The listing builds one solid part. Answer for the finished solid, in the listing's coordinates (mm). Face numbers are marked on the shaded views. A direction names the side the tool comes from. Give positions to 0.01 mm unless a question says otherwise; leave off trailing zeros. Loops run counter-clockwise (first coordinate to the right, second up) from the corner with the lowest first, then second, coordinate; pieces in that order, holes last. Notation, with made-up numbers: M 73.5,36 L 91.5,36 A25 cw 91.5,71 Z; hole C 7,-8 d11. An arc over 180 degrees is marked long. One line per item, written item: value. Start each with the question number.
Q1. The mould has two halves that part along X. Classify the marked faces 6, 7 and 8: +X half, -X half, draft (parallel to the pull), parting line (faces both ways), or undercut.
Q2. Consider L1, parallel to X at y = 7.5, z = 21.5; L2, parallel to Y at x = 8.5, z = 12.5. Determine where each line is inside the solid, lowest interval first.
Q3. For the marked faces 1, 2, 3, 4 and 5, determine the directions among +Z, -Z, +X, -X, +Y, -Y from which every point of the face is accessible in a straight line to the end or side of a thin tool.
Q4. Flat-ended cylindrical pins translate along their axes: pin 1 (8 mm diameter, centred on x = 4, z = 16, fed in from +Y); pin 2 (0.9 mm diameter, centred on x = 18, z = 27.5, fed in from +Y); pin 3 (3.5 mm diameter, centred on x = 1, y = 26.5, fed in from +Z). Find the tip coordinate at first contact, or state that the pin passes through.
Q5. A cutting plane is placed at A-A, the plane y = 16. Determine the outline of the cut face in (x, z), and give its area (3 significant figures).
Q6. A cutting plane is placed at B-B, the plane z = 17.75. Determine the outline of the cut face in (x, y).
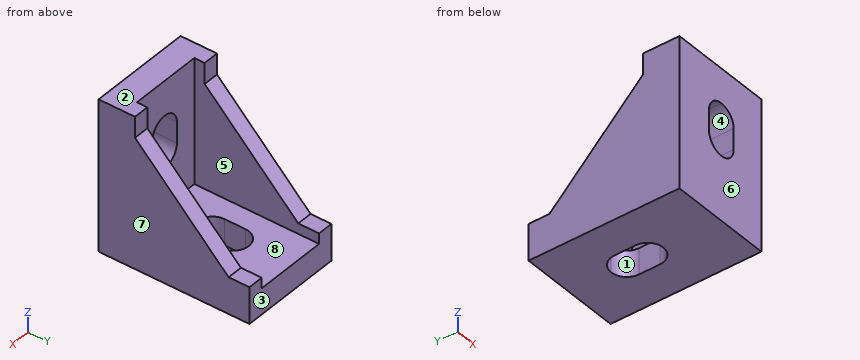
from build123d import *

# Parameters (mm, degrees)
F0_W      = 20
F0_H      = 29
F1_DEPTH  = 5
F3_W      = 20
F3_H      = 24
F4_DEPTH  = 5
F6_DEPTH  = 3
F8_DEPTH  = 3
F9_W      = 6
F9_H      = 10
F10_DEPTH = 29.001
F11_W     = 6
F11_H     = 10
F12_DEPTH = 29.001
F13_R     = 2.99999


# Not quite as in the source:
# - a fillet or chamfer is up to 0.001 mm smaller than in the source, because OpenCascade refuses the exact size


with BuildPart() as f1:
    # F0 (on Top) → F1 (new body)
    with BuildSketch(Plane.XY):
        with Locations((10, 14.5)):
            Rectangle(F0_W, F0_H)
    extrude(amount=F1_DEPTH)

    # F3 (on face) → F4 (join)
    with BuildSketch(Plane.XZ):
        with Locations((10, 17)):
            Rectangle(F3_W, F3_H)
    extrude(amount=-F4_DEPTH)

    # F5 (on face) → F6 (join)
    with BuildSketch(Plane.YZ.offset(20)):
        Polygon((7, 29), (5, 29), (5, 5), (29, 5), (29, 7), (25, 7), (7, 25), align=None)
    extrude(amount=-F6_DEPTH)

    # F7 (on face) → F8 (join)
    with BuildSketch(Plane(origin=(0, 0, 0), x_dir=(0, -1, 0), z_dir=(-1, 0, 0))):
        Polygon((-29, 7), (-29, 5), (-5, 5), (-5, 29), (-7, 29), (-7, 25), (-25, 7), align=None)
    extrude(amount=-F8_DEPTH)

    # F9 (on face) → F10 (cut, through all)
    with BuildSketch(Plane(origin=(0, 0, 0), x_dir=(1, 0, 0), z_dir=(0, 0, -1))):
        with Locations((10, -16)):
            Rectangle(F9_W, F9_H)
    extrude(amount=-F10_DEPTH, mode=Mode.SUBTRACT)

    # F11 (on face) → F12 (cut, through all)
    with BuildSketch(Plane.XZ):
        with Locations((10.2312741801, 17.3546597362)):
            Rectangle(F11_W, F11_H)
    extrude(amount=-F12_DEPTH, mode=Mode.SUBTRACT)

    # F13 (radius 3 in the source; OpenCascade refuses exactly that, so slightly less here)
    f13_edges = [f1.edges().sort_by_distance(p)[0] for p in [
        (7, 11, 2.5),
        (13, 11, 2.5),
        (7, 21, 2.5),
        (13, 21, 2.5),
        (7.231274, 2.5, 12.35466),
        (13.231274, 2.5, 12.35466),
        (7.231274, 2.5, 22.35466),
        (13.231274, 2.5, 22.35466),
    ]]
    fillet(f13_edges, radius=F13_R)


solid = f1.part
Answer block:
1. face 6: draft
1. face 7: +X half
1. face 8: undercut
2. L1: 0 to 3, 17 to 20
2. L2: 0 to 5
3. face 1: +Z, -Z
3. face 2: +Z, +X, -X, +Y, -Y
3. face 3: +Z, -Z, +X, -X, +Y
3. face 4: +Y, -Y
3. face 5: +Z, +Y
4. pin 1: y = 19.87
4. pin 2: y = 7
4. pin 3: z = 7.25
5. outline: M 0,0 L 7,0 L 7,5 L 3,5 L 3,16 L 0,16 Z; M 13,0 L 20,0 L 20,16 L 17,16 L 17,5 L 13,5 Z
5. area: 136 mm^2
6. outline: M 0,0 L 7.23,0 L 7.23,5 L 3,5 L 3,14.25 L 0,14.25 Z; M 13.23,0 L 20,0 L 20,14.25 L 17,14.25 L 17,5 L 13.23,5 Z
